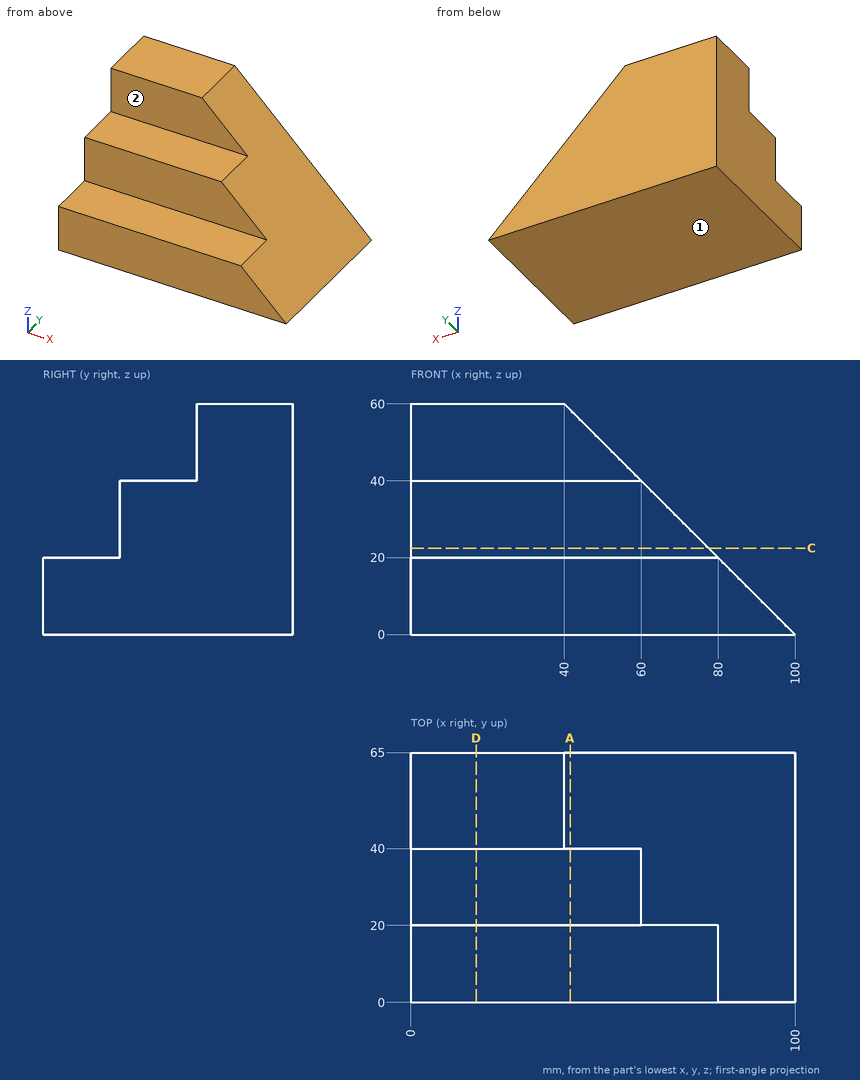
Design review of the part shown in the three views and the two pictorial views. Dimensions are in mm from the part's minimum x, y and z. A direction names the side the tool comes from. Coordinates: 2 decimals unless noted, no trailing zeros. Order: outer loops, then holes, each group sorted by start corner. A loop starts at its lowest first (then second) coordinate and runs counter-clockwise, first axis right, second up.
1) Take a section at D-D, the plane x = 17. Give the boundary of the cut face in (y, z).
2) Clearance check with flat-ended pins moving along their axes: pin 1 (22 mm diameter, centred on x = 16.5, y = 26.5, fed in from +Z); pin 2 (5 mm diameter, centred on y = 41.5, z = 26.5, fed in from +X); pin 3 (3 mm diameter, centred on y = 57.5, z = 39.5, fed in from +X). State where each tip first meets the part, or that it passes through.
3) Take a section at A-A, the plane x = 41.5. Give the boundary of the cut face in (y, z), and give its area (3 significant figures).
4) Wall thickness on line 1 along Y through (x, z) = (21, 44); line 2 along X through (y, z) = (44.5, 40); line 3 along Z through (x, y) = (60, 42): over which ranges is each line inside the solid? List them lowest first.
5) For the marked faces 1 and 2, list the 3-axis set-ups (+Z, -Z, +X, -X, +Y, -Y) from which the entire face can be reached by the end or side of a thin tool; tool diameter is ignored.
6) Take a section at C-C, the plane z = 22.5. Give the boundary of the cut face in (x, y).
Returned:
1. outline: (0, 0) - (65, 0) - (65, 60) - (40, 60) - (40, 40) - (20, 40) - (20, 20) - (0, 20) - close
2. pin 1: stops at z = 40
2. pin 2: stops at x = 76
2. pin 3: stops at x = 62
3. outline: (0, 0) - (65, 0) - (65, 58.5) - (40, 58.5) - (40, 40) - (20, 40) - (20, 20) - (0, 20) - close
3. area: 2,660 mm2
4. line 1: y = 40 to 65
4. line 2: x = 0 to 60
4. line 3: z = 0 to 40
5. face 1: -Z, +X, -X, +Y, -Y
5. face 2: +Z, +X, -X, -Y
6. outline: (0, 20) - (77.5, 20) - (77.5, 65) - (0, 65) - close
